Part print with two shaded views. Sizes in mm from the minimum x, y, z corner. Round coordinates to 2 decimals unless told otherwise and drop trailing zeros. Order: outer loops, then holes, each group sorted by start corner. A loop starts at its lowest first (then second) coordinate and runs counter-clockwise, first axis right, second up. Notation, with made-up numbers: M 43,-36 L 78,-36 A21 cw 78,-29 Z; hole C 59,24 d2. An arc over 180 degrees is marked long. Answer as a JSON object with one key per item and string values.
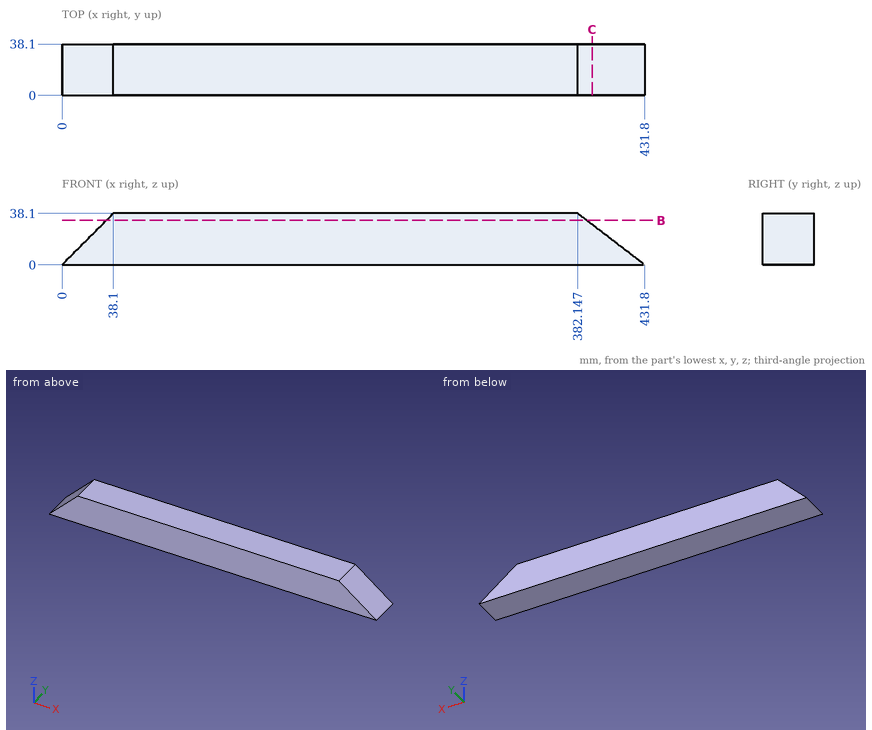
Item 1: Drop a flat-ended pin along its axis: pin 1 Ø2 at (y, z) = (24, 4.5) entering from +X. Give the stop position or say it passes through.
Worked answers:
{"pin 1": "stops at x = 427.24"}
Item 2: Saw through at C-C on x = 393. List the corners of the cut face in (y, z).
Worked answers:
{"outline": "M 0,0 L 38.1,0 L 38.1,29.77 L 0,29.77 Z"}
Item 3: Wall check: line 1 along X through (y, z) = (36, 15); line 2 along X through (y, z) = (24.5, 23) (1 decimal); line 3 along Z through (x, y) = (28, 27.5). Give the ranges that are in metal, low to high. Write a range as [from, to].
Worked answers:
{"line 1": "x = [15, 412.25]", "line 2": "x = [23, 401.8]", "line 3": "z = [0, 28]"}
Item 4: Saw through at B-B on z = 33. List the corners of the cut face in (x, y).
Worked answers:
{"outline": "M 33,0 L 388.79,0 L 388.79,38.1 L 33,38.1 Z"}
